For this review, take the finished solid that the model builds, in its own axes (mm). Face numbers are marked on the shaded views. A direction names the side the tool comes from. Round coordinates to 2 decimals unless told otherwise and drop trailing zeros. Order: outer loops, then holes, each group sorted by start corner. A loop starts at its lowest first (then second) coordinate and runs counter-clockwise, first axis right, second up. Notation, with made-up numbers: (52.25, 77) -> (89.25, 77) arc R8 cw to (89.25, 82) -> close; hole circle Ø5 at (72, -30.5). An arc over 180 degrees is marked (long way). Answer in a Markdown table with one row per item.
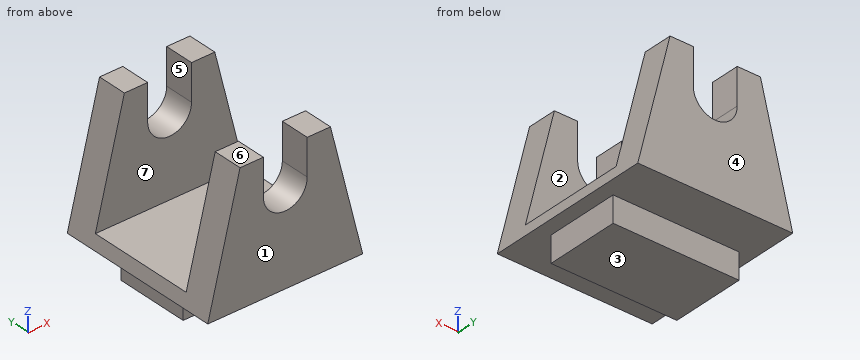
```python
from build123d import *

# Parameters (mm, degrees)
PAD106_DEPTH    = 6.5
SKETCH195_W     = 12
SKETCH195_H     = 9
POCKET046_DEPTH = 4.2
SKETCH196_W     = 9.75
SKETCH196_H     = 5.75
PAD107_DEPTH    = 2


with BuildPart() as part:
    # Sketch194 → Pad106 (new body, symmetric)
    with BuildSketch(Plane.XZ):
        with BuildLine():
            Line((-1.7, 10), (-3.5, 10))
            Line((-3.5, 10), (-6, 0))
            Line((-6, 0), (6, 0))
            Line((6, 0), (3.5, 10))
            Line((3.5, 10), (1.7, 10))
            Line((1.7, 10), (1.7, 7.2))
            ThreePointArc((-1.7, 7.2), (0, 5.5), (1.7, 7.2))
            Line((-1.7, 10), (-1.7, 7.2))
        make_face()
    extrude(amount=PAD106_DEPTH, both=True)

    # Sketch195 → Pocket046 (cut, symmetric)
    with BuildSketch(Plane.XZ):
        with Locations((0, 5.5)):
            Rectangle(SKETCH195_W, SKETCH195_H)
    extrude(amount=POCKET046_DEPTH, both=True, mode=Mode.SUBTRACT)

    # Sketch196 → Pad107 (join)
    with BuildSketch(Plane.XY):
        Rectangle(SKETCH196_W, SKETCH196_H)
    extrude(amount=-PAD107_DEPTH)


with BuildPart() as part_1:
    # Body150 placement: moved
    add(part.part.moved(Location((0, 0, -10))))


solid = part_1.part
```
Q1. Take a section at C-C, the plane z = -2.5. Write out the cut boundary in (x, y) (3 decimals).
Answer key:
| item | result |
|---|---|
| outline | (-4.125, -6.5) -> (-1.7, -6.5) -> (-1.7, -4.2) -> (-4.125, -4.2) -> close; (-4.125, 4.2) -> (-1.7, 4.2) -> (-1.7, 6.5) -> (-4.125, 6.5) -> close; (1.7, -6.5) -> (4.125, -6.5) -> (4.125, -4.2) -> (1.7, -4.2) -> close; (1.7, 4.2) -> (4.125, 4.2) -> (4.125, 6.5) -> (1.7, 6.5) -> close |
Q2. The part is to be moulded in two halves that separate along Y. For the marked faces 1, 2, 3 and 4, say which applies: +Y half, -Y half, draft (parallel to the pull), parting line (faces both ways), or undercut.
Answer key:
| item | result |
|---|---|
| face 1 | -Y half |
| face 2 | undercut |
| face 3 | draft |
| face 4 | +Y half |
Q3. Take a section at A-A, the plane z = -8. Write out the cut boundary in (x, y), then the cut area to 3 significant figures.
Answer key:
| item | result |
|---|---|
| outline | (-5.5, -6.5) -> (5.5, -6.5) -> (5.5, -4.2) -> (-5.5, -4.2) -> close; (-5.5, 4.2) -> (5.5, 4.2) -> (5.5, 6.5) -> (-5.5, 6.5) -> close |
| area | 50.6 mm^2 |
Q4. Take a section at D-D, the plane x = 1.5. Write out the cut boundary in (y, z) (3 decimals).
Answer key:
| item | result |
|---|---|
| outline | (-6.5, -10) -> (-2.875, -10) -> (-2.875, -12) -> (2.875, -12) -> (2.875, -10) -> (6.5, -10) -> (6.5, -3.6) -> (4.2, -3.6) -> (4.2, -9) -> (-4.2, -9) -> (-4.2, -3.6) -> (-6.5, -3.6) -> close |
Q5. Take a section at B-B, the plane y = -1.75. Write out the cut boundary in (x, z) (3 decimals).
Answer key:
| item | result |
|---|---|
| outline | (-6, -10) -> (-4.875, -10) -> (-4.875, -12) -> (4.875, -12) -> (4.875, -10) -> (6, -10) -> (5.75, -9) -> (-5.75, -9) -> close |
Q6. Clearance check with flat-ended pins moving along their axes: pin 1 Ø1.8 at (y, z) = (5.5, -1.5) entering from +X; pin 2 Ø0.6 at (y, z) = (-0.5, -11) entering from -X (3 decimals); pin 3 Ø4 at (y, z) = (1.5, -5) entering from -X; pin 4 Ø1.8 at (y, z) = (-5.5, -2) entering from +X (3 decimals). State where each tip first meets the part, or that it passes through.
Answer key:
| item | result |
|---|---|
| pin 1 | stops at x = 4.1 |
| pin 2 | stops at x = -4.875 |
| pin 3 | passes through |
| pin 4 | stops at x = 4.225 |
Q7. Tool access review of the marked faces 5, 6 and 7: name each direction out of +Z, -Z, +X, -X, +Y, -Y from which nothing blocks a thin tool from reaching the whole face with its end or side.
Answer key:
| item | result |
|---|---|
| face 5 | +Z, +Y, -Y |
| face 6 | +Z, +X, -X, +Y, -Y |
| face 7 | +Z, +X, -X |
Q8. To check wall thickness, follow probe 1 along Y at (x, z) = (2, -2.5); probe 2 along Z at (x, y) = (-3, -3.25); probe 3 along Z at (x, y) = (1.25, -2). State the ranges of each line that lie inside material, in increasing order.
Answer key:
| item | result |
|---|---|
| probe 1 | y = -6.5 to -4.2, 4.2 to 6.5 |
| probe 2 | z = -10 to -9 |
| probe 3 | z = -12 to -9 |
